from build123d import *

# Parameters (mm, degrees)
SKETCH1_W            = 300
SKETCH1_H            = 20
BOSS_EXTRUDE1_DEPTH  = 8
SKETCH2_W            = 34
SKETCH2_H            = 8
BOSS_EXTRUDE2_DEPTH  = 9
SKETCH3_W            = 34
SKETCH3_H            = 8
BOSS_EXTRUDE3_DEPTH  = 9
SKETCH4_R            = 1.45
CUT_EXTRUDE1_DEPTH   = 302.504560496
SKETCH5_W            = 25
SKETCH5_H            = 8
BOSS_EXTRUDE4_DEPTH  = 17
SKETCH6_W            = 25
SKETCH6_H            = 8
BOSS_EXTRUDE5_DEPTH  = 17
SKETCH7_W            = 10
SKETCH7_H            = 38
CUT_EXTRUDE2_DEPTH   = 303.37890138
SKETCH8_W            = 7
SKETCH8_H            = 16
CUT_EXTRUDE3_DEPTH   = 4
CUT_EXTRUDE4_DEPTH   = 7
BOSS_EXTRUDE6_DEPTH  = 10
SKETCH12_W           = 8
SKETCH12_H           = 8
BOSS_EXTRUDE7_DEPTH  = 17
SKETCH13_R           = 1.7
CUT_EXTRUDE6_DEPTH   = 305.926220585
SKETCH14_W           = 20
SKETCH14_H           = 13
BOSS_EXTRUDE8_DEPTH  = 12
SKETCH15_R           = 1.6
CUT_EXTRUDE7_DEPTH   = 20
SKETCH16_W           = 20
SKETCH16_H           = 13
BOSS_EXTRUDE9_DEPTH  = 12
SKETCH17_R           = 1.6
CUT_EXTRUDE8_DEPTH   = 20
SKETCH18_W           = 20
SKETCH18_H           = 13
BOSS_EXTRUDE10_DEPTH = 12
CUT_EXTRUDE9_START   = -20
SKETCH19_R           = 1.6
CUT_EXTRUDE9_DEPTH   = 20
SKETCH20_W           = 20
SKETCH20_H           = 13
BOSS_EXTRUDE11_DEPTH = 12
CUT_EXTRUDE10_START  = -20
SKETCH21_R           = 1.6
CUT_EXTRUDE10_DEPTH  = 20
SKETCH22_W           = 207
SKETCH22_H           = 50
BOSS_EXTRUDE12_DEPTH = 8
SKETCH23_W           = 191
SKETCH23_H           = 44
CUT_EXTRUDE11_DEPTH  = 4
SKETCH24_W           = 10
SKETCH24_H           = 44
BOSS_EXTRUDE14_DEPTH = 19.4
SKETCH25_R           = 1.45
CUT_EXTRUDE12_DEPTH  = 15
FILLET1_R            = 5
FILLET2_R            = 5
FILLET3_R            = 8
FILLET4_R            = 15
FILLET5_R            = 25
FILLET6_R            = 3
SKETCH27_W           = 1.8
SKETCH27_H           = 5
CUT_EXTRUDE13_DEPTH  = 19.4


with BuildPart() as part:
    # Sketch1 → Boss-Extrude1 (new body)
    with BuildSketch(Plane(origin=(0, 0, 0), x_dir=(1, 0, 0), z_dir=(0, 1, 0))):
        with Locations((150, -10)):
            Rectangle(SKETCH1_W, SKETCH1_H)
    extrude(amount=BOSS_EXTRUDE1_DEPTH)

    # Sketch2 → Boss-Extrude2 (add)
    with BuildSketch(Plane.XY.offset(20)):
        with Locations((17, 4)):
            Rectangle(SKETCH2_W, SKETCH2_H)
        with Locations((283, 4)):
            Rectangle(SKETCH2_W, SKETCH2_H)
    extrude(amount=BOSS_EXTRUDE2_DEPTH)

    # Sketch3 → Boss-Extrude3 (add)
    with BuildSketch(Plane(origin=(0, 0, 0), x_dir=(-1, 0, 0), z_dir=(0, 0, -1))):
        with Locations((-17, 4)):
            Rectangle(SKETCH3_W, SKETCH3_H)
        with Locations((-283, 4)):
            Rectangle(SKETCH3_W, SKETCH3_H)
    extrude(amount=BOSS_EXTRUDE3_DEPTH)

    # Sketch4 → Cut-Extrude1 (cut, through all)
    with BuildSketch(Plane(origin=(0, 8, 0), x_dir=(1, 0, 0), z_dir=(0, 1, 0))):
        with Locations(Location((4, 5, 0), (0, 0, 270))):
            Circle(SKETCH4_R)
        with Locations(Location((30, 5, 0), (0, 0, 270))):
            Circle(SKETCH4_R)
        with Locations(Location((30, -25, 0), (0, 0, 270))):
            Circle(SKETCH4_R)
        with Locations(Location((4, -25, 0), (0, 0, 270))):
            Circle(SKETCH4_R)
        with Locations(Location((296, -25, 0), (0, 0, 270))):
            Circle(SKETCH4_R)
        with Locations(Location((296, 5, 0), (0, 0, 270))):
            Circle(SKETCH4_R)
        with Locations(Location((270, -25, 0), (0, 0, 270))):
            Circle(SKETCH4_R)
        with Locations(Location((270, 5, 0), (0, 0, 270))):
            Circle(SKETCH4_R)
    extrude(amount=-CUT_EXTRUDE1_DEPTH, mode=Mode.SUBTRACT)

    # Sketch5 → Boss-Extrude4 (add)
    with BuildSketch(Plane.XY.offset(20)):
        with Locations((253.5, 4)):
            Rectangle(SKETCH5_W, SKETCH5_H)
    extrude(amount=BOSS_EXTRUDE4_DEPTH)

    # Sketch6 → Boss-Extrude5 (add)
    with BuildSketch(Plane(origin=(0, 0, 0), x_dir=(-1, 0, 0), z_dir=(0, 0, -1))):
        with Locations((-253.5, 4)):
            Rectangle(SKETCH6_W, SKETCH6_H)
    extrude(amount=BOSS_EXTRUDE5_DEPTH)

    # Sketch7 → Cut-Extrude2 (cut, through all)
    with BuildSketch(Plane(origin=(0, 8, 0), x_dir=(1, 0, 0), z_dir=(0, 1, 0))):
        with Locations((254, -10)):
            Rectangle(SKETCH7_W, SKETCH7_H)
    extrude(amount=-CUT_EXTRUDE2_DEPTH, mode=Mode.SUBTRACT)

    # Sketch8 → Cut-Extrude3 (cut)
    with BuildSketch(Plane(origin=(0, 8, 0), x_dir=(1, 0, 0), z_dir=(0, 1, 0))):
        with Locations((262.5, -10)):
            Rectangle(SKETCH8_W, SKETCH8_H)
    extrude(amount=-CUT_EXTRUDE3_DEPTH, mode=Mode.SUBTRACT)

    # Sketch9 → Cut-Extrude4 (cut)
    with BuildSketch(Plane.ZY.offset(-259)):
        Polygon((18, 4), (22, 8), (18, 8), align=None)
        Polygon((2, 4), (-2, 8), (2, 8), align=None)
    extrude(amount=-CUT_EXTRUDE4_DEPTH, mode=Mode.SUBTRACT)

    # Sketch10 → Boss-Extrude6 (add)
    with BuildSketch(Plane.ZY.offset(-259)):
        Polygon((-2, 0), (-9, 8), (-9, 0), align=None)
        Polygon((29, 8), (22, 0), (29, 0), align=None)
    extrude(amount=BOSS_EXTRUDE6_DEPTH)

    # Sketch12 → Boss-Extrude7 (add)
    with BuildSketch(Plane.XY.offset(37)):
        with Locations((245, 4)):
            Rectangle(SKETCH12_W, SKETCH12_H)
    extrude(amount=BOSS_EXTRUDE7_DEPTH)

    # Sketch13 → Cut-Extrude6 (cut, through all)
    with BuildSketch(Plane(origin=(0, 8, 0), x_dir=(1, 0, 0), z_dir=(0, 1, 0))):
        with Locations(Location((245, -50, 0), (0, 0, 270))):
            Circle(SKETCH13_R)
        with Locations(Location((245, -18, 0), (0, 0, 270))):
            Circle(SKETCH13_R)
    extrude(amount=-CUT_EXTRUDE6_DEPTH, mode=Mode.SUBTRACT)

    # Sketch14 → Boss-Extrude8 (add)
    with BuildSketch(Plane.XY.offset(29)):
        with Locations((285, 6.5)):
            Rectangle(SKETCH14_W, SKETCH14_H)
    extrude(amount=BOSS_EXTRUDE8_DEPTH)

    # Sketch15 → Cut-Extrude7 (cut)
    with BuildSketch(Plane(origin=(295, 0, 0), x_dir=(0, 0, -1), z_dir=(1, 0, 0))):
        with Locations((-35, 8)):
            Circle(SKETCH15_R)
    extrude(amount=-CUT_EXTRUDE7_DEPTH, mode=Mode.SUBTRACT)

    # Sketch16 → Boss-Extrude9 (add)
    with BuildSketch(Plane(origin=(0, 0, -9), x_dir=(-1, 0, 0), z_dir=(0, 0, -1))):
        with Locations((-285, 6.5)):
            Rectangle(SKETCH16_W, SKETCH16_H)
    extrude(amount=BOSS_EXTRUDE9_DEPTH)

    # Sketch17 → Cut-Extrude8 (cut)
    with BuildSketch(Plane(origin=(295, 0, 0), x_dir=(0, 0, -1), z_dir=(1, 0, 0))):
        with Locations((15, 8)):
            Circle(SKETCH17_R)
    extrude(amount=-CUT_EXTRUDE8_DEPTH, mode=Mode.SUBTRACT)

    # Sketch18 → Boss-Extrude10 (add)
    with BuildSketch(Plane(origin=(0, 0, -9), x_dir=(-1, 0, 0), z_dir=(0, 0, -1))):
        with Locations((-15, 6.5)):
            Rectangle(SKETCH18_W, SKETCH18_H)
    extrude(amount=BOSS_EXTRUDE10_DEPTH)

    # Sketch19 → Cut-Extrude9 (cut)
    with BuildSketch(Plane.ZY.offset(-5).offset(CUT_EXTRUDE9_START)):
        with Locations(Location((-15, 8, 0), (0, 0, 180))):
            Circle(SKETCH19_R)
    extrude(amount=CUT_EXTRUDE9_DEPTH, mode=Mode.SUBTRACT)

    # Sketch20 → Boss-Extrude11 (add)
    with BuildSketch(Plane.XY.offset(29)):
        with Locations((15, 6.5)):
            Rectangle(SKETCH20_W, SKETCH20_H)
    extrude(amount=BOSS_EXTRUDE11_DEPTH)

    # Sketch21 → Cut-Extrude10 (cut)
    with BuildSketch(Plane.ZY.offset(-5).offset(CUT_EXTRUDE10_START)):
        with Locations(Location((35, 8, 0), (0, 0, 180))):
            Circle(SKETCH21_R)
    extrude(amount=CUT_EXTRUDE10_DEPTH, mode=Mode.SUBTRACT)

    # Sketch22 → Boss-Extrude12 (add)
    with BuildSketch(Plane(origin=(0, 0, 0), x_dir=(-1, 0, 0), z_dir=(0, -1, 0))):
        with Locations((-137.5, -45)):
            Rectangle(SKETCH22_W, SKETCH22_H)
        with Locations((-137.5, 25)):
            Rectangle(SKETCH22_W, SKETCH22_H)
    extrude(amount=-BOSS_EXTRUDE12_DEPTH)

    # Sketch23 → Cut-Extrude11 (cut)
    with BuildSketch(Plane(origin=(0, 8, 0), x_dir=(1, 0, 0), z_dir=(0, 1, 0))):
        with Locations((137.5, -42)):
            Rectangle(SKETCH23_W, SKETCH23_H)
        with Locations((137.5, 22)):
            Rectangle(SKETCH23_W, SKETCH23_H)
    extrude(amount=-CUT_EXTRUDE11_DEPTH, mode=Mode.SUBTRACT)

    # Sketch24 → Boss-Extrude14 (add)
    with BuildSketch(Plane(origin=(0, 4, 0), x_dir=(1, 0, 0), z_dir=(0, 1, 0))):
        with Locations((103.4, -42)):
            Rectangle(SKETCH24_W, SKETCH24_H)
        with Locations((52, -42)):
            Rectangle(SKETCH24_W, SKETCH24_H)
    extrude(amount=BOSS_EXTRUDE14_DEPTH)

    # Sketch25 → Cut-Extrude12 (cut)
    with BuildSketch(Plane(origin=(0, 23.4, 0), x_dir=(1, 0, 0), z_dir=(0, 1, 0))):
        with Locations(Location((102.6, -49, 0), (0, 0, 270))):
            Circle(SKETCH25_R)
        with Locations(Location((102.6, -39, 0), (0, 0, 270))):
            Circle(SKETCH25_R)
        with Locations(Location((52.8, -49, 0), (0, 0, 270))):
            Circle(SKETCH25_R)
        with Locations(Location((52.8, -39, 0), (0, 0, 270))):
            Circle(SKETCH25_R)
    extrude(amount=-CUT_EXTRUDE12_DEPTH, mode=Mode.SUBTRACT)

    # Fillet1
    fillet1_edges = [part.edges().sort_by_distance(p)[0] for p in [
        (103.4, 8, 64),
        (103.4, 8, 20),
        (52, 8, 64),
        (52, 8, 20),
    ]]
    fillet(fillet1_edges, radius=FILLET1_R)

    # Fillet2
    fillet2_edges = [part.edges().sort_by_distance(p)[0] for p in [
        (47, 4, 42),
        (108.4, 4, 42),
    ]]
    fillet(fillet2_edges, radius=FILLET2_R - 0.0001)  # a hair under: the kernel refuses the full size

    # Fillet3
    fillet3_edges = [part.edges().sort_by_distance(p)[0] for p in [
        (241, 4, 54),
    ]]
    fillet(fillet3_edges, radius=FILLET3_R - 0.0001)  # a hair under: the kernel refuses the full size

    # Fillet4
    fillet4_edges = [part.edges().sort_by_distance(p)[0] for p in [
        (249, 4, 37),
    ]]
    fillet(fillet4_edges, radius=FILLET4_R)

    # Fillet5
    fillet5_edges = [part.edges().sort_by_distance(p)[0] for p in [
        (241, 4, -17),
    ]]
    fillet(fillet5_edges, radius=FILLET5_R - 0.0001)  # a hair under: the kernel refuses the full size

    # Fillet6
    fillet6_edges = [part.edges().sort_by_distance(p)[0] for p in [
        (285, 13, 29),
        (285, 13, 41),
        (285, 13, -9),
        (285, 13, -21),
        (15, 13, -9),
        (15, 13, -21),
        (15, 13, 29),
        (15, 13, 41),
    ]]
    fillet(fillet6_edges, radius=FILLET6_R)

    # Sketch27 → Cut-Extrude13 (cut)
    with BuildSketch(Plane(origin=(0, 23.4, 0), x_dir=(1, 0, 0), z_dir=(0, 1, 0))):
        with Locations((56.1, -44.5)):
            Rectangle(SKETCH27_W, SKETCH27_H)
        with Locations((99.3, -44.5)):
            Rectangle(SKETCH27_W, SKETCH27_H)
    extrude(amount=-CUT_EXTRUDE13_DEPTH, mode=Mode.SUBTRACT)


solid = part.part
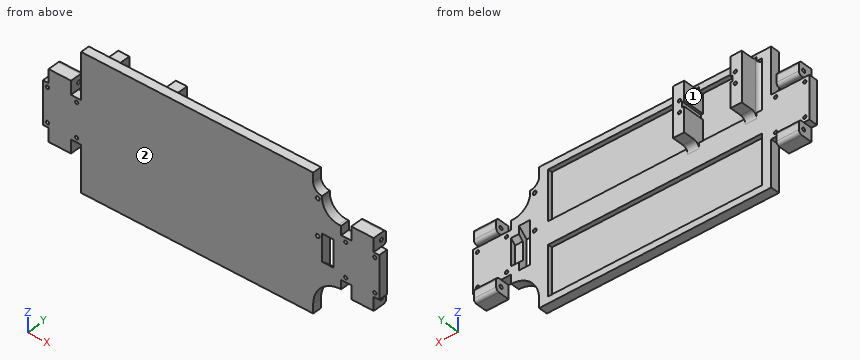
Design review of the part built by this model. Coordinates are the model's own, in mm. Face numbers are marked on the shaded views. Round coordinates to 2 decimals unless told otherwise and drop trailing zeros. Write each loop counter-clockwise with the first axis right and the second up, starting at its lowest first coordinate (ties: lowest second). Pieces come first, ordered by that corner, then holes. Notation, with made-up numbers: (31, 15.5) -> (45, 15.5) arc R20 cw to (45, 27.5) -> close; hole circle Ø1 at (40.25, 41.5). An arc over 180 degrees is marked (long way). One line per item, written item: value. Start each with the question number.
Q1. Add section B-B (z = -29). Give the boundary of the cut face in (x, y), then the cut area to 3 significant figures.
Q2. To check wall thickness, follow probe 1 along Z at (x, y) = (270, 4.5); probe 2 along Z at (x, y) = (226.5, 4.75); probe 3 along Z at (x, y) = (278.5, 8.75). State the ranges of each line that lie inside material, in increasing order.
Q3. Insertion check: P1, Ø0.6, axis at x = 280.5, y = 9, coming from the -Z side; P2, Ø6, axis at y = 18, z = 30, coming from the +X side; P3, Ø2.5, axis at y = 8, z = -15, coming from the -X side; P4, Ø1.5, axis at x = 184.5, z = -3.5, coming from the -Y side. Each pin has a flat end and moves straight along its axis. Give the tip position at first contact, or say it passes through.
Q4. The part is to be moulded in two halves that separate along X. For the marked faces 1 and 2, say which applies: pulls with the +X half, pulls with the -X half, needs draft (parallel to the pull), parting line crosses it, or undercut.
Q5. Add section A-A (x = 229). Give the boundary of the cut face in (y, z).
Response:
1. outline: (34, 0) -> (244.65, 0) -> (244.65, 8) -> (233, 8) -> (233, 4) -> (42, 4) -> (42, 8) -> (34, 8) -> close
1. area: 921 mm^2
2. probe 1: z = -9 to -6.45, -3.55 to 23.55, 26.45 to 29
2. probe 2: z = -50 to -44, 0 to 20, 64 to 70
2. probe 3: z = -21 to -16.41, -13.59 to -9, 29 to 33.59, 36.41 to 41
3. P1: stops at z = -21
3. P2: stops at x = 108.4
3. P3: stops at x = 34
3. P4: stops at y = 0
4. face 1: undercut
4. face 2: needs draft
5. outline: (0, -50) -> (8, -50) -> (8, -44) -> (4, -44) -> (4, 0) -> (8, 0) -> (8, 20) -> (4, 20) -> (4, 64) -> (8, 64) -> (8, 70) -> (0, 70) -> close
